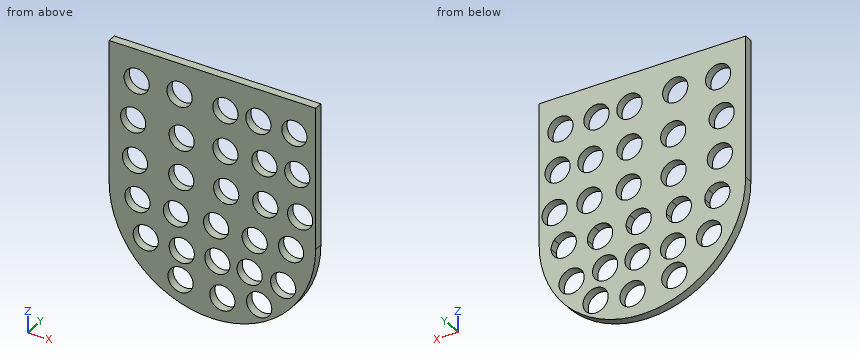
from build123d import *

# Parameters (mm, degrees)
F0_R     = 7.5
F1_DEPTH = 5


with BuildPart() as f1:
    # F0 (on Front) → F1 (new body)
    with BuildSketch(Plane.XZ):
        with BuildLine():
            Line((-86.710327, 94.337149), (-86.710327, 10.077905))
            Line((-86.710327, 10.077905), (-75.277857, 10.077905))
            ThreePointArc((-75.277857, 10.077905), (-69.84026, 12.412391), (-64.402663, 10.077905))
            Line((-64.402663, 10.077905), (-51.199337, 10.077905))
            ThreePointArc((-51.199337, 10.077905), (-46.909187, 11.426107), (-42.619037, 10.077905))
            Line((-42.619037, 10.077905), (-28.184067, 10.077905))
            ThreePointArc((-28.184067, 10.077905), (-22.991827, 12.165822), (-17.799587, 10.077905))
            Line((-17.799587, 10.077905), (-3.477754, 10.077905))
            ThreePointArc((-3.477754, 10.077905), (0, 10.932965), (3.477754, 10.077905))
            Line((3.477754, 10.077905), (15.975848, 10.077905))
            ThreePointArc((15.975848, 10.077905), (21.637471, 12.65896), (27.299095, 10.077905))
            Line((27.299095, 10.077905), (36.289673, 10.077905))
            Line((36.289673, 10.077905), (36.289673, 94.337149))
            Line((36.289673, 94.337149), (-86.710327, 94.337149))
        make_face()
        with Locations((-71.317263, 27.843174)):
            Circle(F0_R, mode=Mode.SUBTRACT)
        with Locations((-72.399746, 51.555946)):
            Circle(F0_R, mode=Mode.SUBTRACT)
        with Locations((-43.777015, 26.649399)):
            Circle(F0_R, mode=Mode.SUBTRACT)
        with Locations((-43.526709, 50.178468)):
            Circle(F0_R, mode=Mode.SUBTRACT)
        with Locations((-70.309795, 75.459704)):
            Circle(F0_R, mode=Mode.SUBTRACT)
        with Locations((-44.778254, 75.960323)):
            Circle(F0_R, mode=Mode.SUBTRACT)
        with Locations((-16.993923, 27.150016)):
            Circle(F0_R, mode=Mode.SUBTRACT)
        with Locations((-17.494541, 50.929397)):
            Circle(F0_R, mode=Mode.SUBTRACT)
        with Locations((6.284834, 26.899708)):
            Circle(F0_R, mode=Mode.SUBTRACT)
        with Locations((27.060509, 26.399089)):
            Circle(F0_R, mode=Mode.SUBTRACT)
        with Locations((5.784216, 51.179707)):
            Circle(F0_R, mode=Mode.SUBTRACT)
        with Locations((25.308343, 51.179707)):
            Circle(F0_R, mode=Mode.SUBTRACT)
        with Locations((-17.494541, 75.209394)):
            Circle(F0_R, mode=Mode.SUBTRACT)
        with Locations((2.142422, 75.247116)):
            Circle(F0_R, mode=Mode.SUBTRACT)
        with Locations((23.602774, 75.152084)):
            Circle(F0_R, mode=Mode.SUBTRACT)
        with BuildLine():
            Line((-75.277857, 10.077905), (-86.710327, 10.077905))
            ThreePointArc((-86.710327, 10.077905), (-25.210327, -51.422095), (36.289673, 10.077905))
            Line((36.289673, 10.077905), (27.299095, 10.077905))
            ThreePointArc((27.299095, 10.077905), (28.66286, 7.784586), (29.137471, 5.15896))
            ThreePointArc((29.137471, 5.15896), (19.011845, -1.866429), (15.975848, 10.077905))
            Line((15.975848, 10.077905), (3.477754, 10.077905))
            ThreePointArc((3.477754, 10.077905), (6.416119, 7.316703), (7.5, 3.432965))
            ThreePointArc((7.5, 3.432965), (-3.883738, -2.983154), (-3.477754, 10.077905))
            Line((-3.477754, 10.077905), (-17.799587, 10.077905))
            ThreePointArc((-17.799587, 10.077905), (-16.092849, 7.607607), (-15.491827, 4.665822))
            ThreePointArc((-15.491827, 4.665822), (-25.933612, -2.233156), (-28.184067, 10.077905))
            Line((-28.184067, 10.077905), (-42.619037, 10.077905))
            ThreePointArc((-42.619037, 10.077905), (-40.259897, 7.395536), (-39.409187, 3.926107))
            ThreePointArc((-39.409187, 3.926107), (-50.378616, -2.723183), (-51.199337, 10.077905))
            Line((-51.199337, 10.077905), (-64.402663, 10.077905))
            ThreePointArc((-64.402663, 10.077905), (-62.874918, 7.6934), (-62.34026, 4.912391))
            ThreePointArc((-62.34026, 4.912391), (-72.621269, -2.052951), (-75.277857, 10.077905))
        make_face()
        with Locations((-64.908847, -16.292689)):
            Circle(F0_R, mode=Mode.SUBTRACT)
        with Locations((-44.196907, -34.538925)):
            Circle(F0_R, mode=Mode.SUBTRACT)
        with Locations((-43.457195, -16.785832)):
            Circle(F0_R, mode=Mode.SUBTRACT)
        with Locations((-19.293265, -37.251204)):
            Circle(F0_R, mode=Mode.SUBTRACT)
        with Locations((2.651528, -34.045782)):
            Circle(F0_R, mode=Mode.SUBTRACT)
        with Locations((-22.252114, -16.292689)):
            Circle(F0_R, mode=Mode.SUBTRACT)
        with Locations((-3.019601, -16.539263)):
            Circle(F0_R, mode=Mode.SUBTRACT)
        with Locations((16.95263, -17.772116)):
            Circle(F0_R, mode=Mode.SUBTRACT)
    extrude(amount=F1_DEPTH)


solid = f1.part
Here's how the part is built. I have some questions about the finished solid (model axes, mm). Coordinates: 2 decimals unless noted, no trailing zeros. Order: outer loops, then holes, each group sorted by start corner. A loop starts at its lowest first (then second) coordinate and runs counter-clockwise, first axis right, second up. Notation, with made-up numbers: (-12, 78.25) -> (44, 78.25) arc R16 cw to (44, 109.25) -> close; hole circle Ø8 at (-11, 31). An arc over 180 degrees is marked (long way). Answer in a Markdown table with one row per item.
(1) I want a section at C-C on z = -40. List the corners of the cut face in (x, y) for me.
Answer key:
| item | result |
|---|---|
| outline | (-60.91, -5) -> (-49.34, -5) -> (-49.34, 0) -> (-60.91, 0) -> close; (-39.06, -5) -> (-26.27, -5) -> (-26.27, 0) -> (-39.06, 0) -> close; (-12.32, -5) -> (-1.91, -5) -> (-1.91, 0) -> (-12.32, 0) -> close; (7.21, -5) -> (10.49, -5) -> (10.49, 0) -> (7.21, 0) -> close |
(2) I want a section at B-B on z = 23. List the corners of the cut face in (x, y) for me, then the cut area to 3 significant figures.
Answer key:
| item | result |
|---|---|
| outline | (-86.71, -5) -> (-77.04, -5) -> (-77.04, 0) -> (-86.71, 0) -> close; (-65.59, -5) -> (-50.33, -5) -> (-50.33, 0) -> (-65.59, 0) -> close; (-37.22, -5) -> (-23.24, -5) -> (-23.24, 0) -> (-37.22, 0) -> close; (-10.75, -5) -> (-0.12, -5) -> (-0.12, 0) -> (-10.75, 0) -> close; (12.69, -5) -> (20.37, -5) -> (20.37, 0) -> (12.69, 0) -> close; (33.75, -5) -> (36.29, -5) -> (36.29, 0) -> (33.75, 0) -> close |
| area | 299 mm^2 |
(3) I want a section at A-A on x = -69. List the corners of the cut face in (y, z) for me.
Answer key:
| item | result |
|---|---|
| outline | (-5, -33.1) -> (0, -33.1) -> (0, -22.58) -> (-5, -22.58) -> close; (-5, -10.01) -> (0, -10.01) -> (0, -2.54) -> (-5, -2.54) -> close; (-5, 12.37) -> (0, 12.37) -> (0, 20.71) -> (-5, 20.71) -> close; (-5, 34.98) -> (0, 34.98) -> (0, 44.87) -> (-5, 44.87) -> close; (-5, 58.24) -> (0, 58.24) -> (0, 68.07) -> (-5, 68.07) -> close; (-5, 82.84) -> (0, 82.84) -> (0, 94.34) -> (-5, 94.34) -> close |
(4) Will these pins go through, and if not, where does the flat tip stop? pin 1 Ø2 at (y, z) = (-3.5, 4.5) entering from +X; pin 2 Ø1.5 at (x, y) = (-24.5, -1) entering from -Z.
Answer key:
| item | result |
|---|---|
| pin 1 | x = 36.12 |
| pin 2 | z = -51.42 |
(5) Please list where these lines run through material, in increasing order: probe 1 along X at (y, z) = (-1, -37.5); probe 2 along Z at (x, y) = (-2.5, -1.7); probe 3 along Z at (x, y) = (-74, -2.6).
Answer key:
| item | result |
|---|---|
| probe 1 | -64.18 to -51.09, -37.31 to -26.79, -11.8 to -4.01, 9.31 to 13.76 |
| probe 2 | -47.08 to -39.5, -28.59 to -24.02, -9.06 to -3.64, 10.5 to 69.36, 81.14 to 94.34 |
| probe 3 | -27.36 to -1.33, 11.15 to 20.84, 34.85 to 44.23, 58.88 to 68.93, 81.99 to 94.34 |
(6) I want a section at D-D on y = -3.65. Count the separate pieces of the cut face and the enclosed holes in it, then the cut area to 3 significant figures.
Answer key:
| item | result |
|---|---|
| separate pieces | 1 |
| enclosed holes | 28 |
| area | 11,400 mm^2 |
